The figure shows three views and two pictorial views of one solid part (mm, origin at its lowest corner). Answer the questions. Coordinates: 2 decimals unless noted, no trailing zeros. Write each loop counter-clockwise with the first axis right and the second up, starting at its lowest first coordinate (ties: lowest second). Pieces come first, ordered by that corner, then holes. Notation, with made-up numbers: M 20,84 L 72,84 A13 cw 72,100 Z; hole C 15,-36 d10. An arc over 180 degrees is marked long. Use CSV: the item, a comma, the result in double quotes.
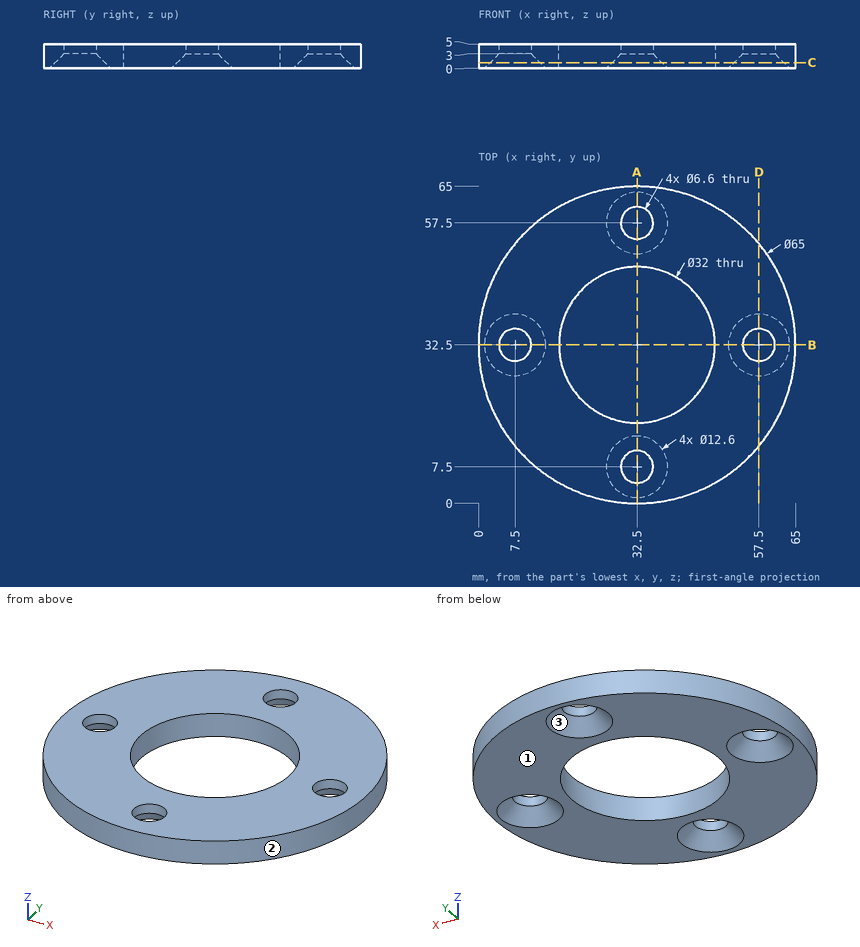
Item 1: Consider probe 1 along X at (y, z) = (29.5, 0.25); probe 2 along Y at (x, z) = (32.5, 1.55); probe 3 along Y at (x, z) = (31.5, 3.15). Determine where each line is inside the solid, lowest interval first.
Answer:
probe 1,"x = 0.14 to 2.25, 12.75 to 16.78, 48.22 to 52.25, 62.75 to 64.86"
probe 2,"y = 0 to 2.75, 12.25 to 16.5, 48.5 to 52.75, 62.25 to 65"
probe 3,"y = 0.02 to 4.36, 10.64 to 16.53, 48.47 to 54.36, 60.64 to 64.98"
Item 2: The part is cut by section D-D (x = 57.5). Write down the section's boundary in (y, z), then the cut area to 3 significant figures.
Answer:
outline,"M 11.73,0 L 26.2,0 L 29.2,3 L 29.2,5 L 11.73,5 Z; M 35.8,3 L 38.8,0 L 53.27,0 L 53.27,5 L 35.8,5 Z"
area,"166 mm2"
Item 3: For a pull along Y with two mould halves and no side action, classify the marked faces 1, 2 and 3 as released by +Y, released by -Y, zero draft, split by the parting line, or undercut.
Answer:
face 1,"zero draft"
face 2,"split by the parting line"
face 3,"undercut"
Item 4: Given pin 1 (2 mm diameter, centred on x = 26.5, z = 1, fed in from -Y); pin 2 (1.5 mm diameter, centred on x = 36, y = 10, fed in from -Z); pin 3 (4 mm diameter, centred on x = 32.5, y = 57.5, fed in from +Z); pin 4 (8.5 mm diameter, centred on x = 7.5, y = 32.5, fed in from -Z), each flat-ended and moving along its own axis, determine where each tip first touches the part or whether it passes through.
Answer:
pin 1,"stops at y = 0.39"
pin 2,"stops at z = 1.25"
pin 3,"passes through"
pin 4,"stops at z = 2.05"
Item 5: The part is cut by section A-A (x = 32.5). Write down the section's boundary in (y, z).
Answer:
outline,"M 0,0 L 1.2,0 L 4.2,3 L 4.2,5 L 0,5 Z; M 10.8,3 L 13.8,0 L 16.5,0 L 16.5,5 L 10.8,5 Z; M 48.5,0 L 51.2,0 L 54.2,3 L 54.2,5 L 48.5,5 Z; M 60.8,3 L 63.8,0 L 65,0 L 65,5 L 60.8,5 Z"
Item 6: The part is cut by section C-C (z = 1.2). Write down the section's boundary in (x, y).
Answer:
outline,"C 32.5,32.5 d65; hole C 7.5,32.5 d10.2; hole C 32.5,32.5 d32; hole C 32.5,7.5 d10.2; hole C 32.5,57.5 d10.2; hole C 57.5,32.5 d10.2"
